from build123d import *

# Parameters (mm, degrees)
HEX_2_DEPTH = 4.7


with BuildPart() as part:
    # BodySketch → BaseBody (revolve)
    with BuildSketch(Plane(origin=(0, 0, 0), x_dir=(1, 0, 0), z_dir=(0, 1, 0)), mode=Mode.PRIVATE) as basebody_sk:
        Polygon((79.3095, 4), (80, 3.3095), (80, 0), (-0.6, 0), (-0.6, 6.5), (0, 6.5), (0, 4), align=None)
    revolve(basebody_sk.sketch.rotate(Axis((0, 0, 0), (1, 0, 0)), 180), axis=Axis((0, 0, 0), (1, 0, 0)))

    # HeadSketch → Hex 2 (add)
    with BuildSketch(Plane.ZY.offset(0.6)):
        Polygon((7.505553499, 0), (3.75277675, 6.5), (-3.75277675, 6.5), (-7.505553499, 0), (-3.75277675, -6.5), (3.75277675, -6.5), align=None)
    extrude(amount=HEX_2_DEPTH)


solid = part.part
Could you check a few things on this model? Use its own coordinates, in mm. A direction names the side the tool comes from. Coordinates: 2 decimals unless noted, no trailing zeros. Write each loop counter-clockwise with the first axis right and the second up, starting at its lowest first coordinate (ties: lowest second). Pieces come first, ordered by that corner, then holes. Notation, with made-up numbers: M -24.5,27 L 3.5,27 A21 ccw 3.5,59 Z; hole C 85,27.25 d2. An arc over 180 degrees is marked long. One line per question, with ' | ' between items.
1) I need wall thicknesses on probe 1 along X at (y, z) = (-5.25, -3); probe 2 along X at (y, z) = (-5.25, -4); probe 3 along Y at (x, z) = (4, -2). Which ranges of each line are inside material? Lowest first, please. Write a range as [from, to].
Checks:
probe 1: [-5.3, 0] | probe 2: [-5.3, -0.6] | probe 3: [-3.46, 3.46]
2) For pin 1 Ø3.5 at (y, z) = (4.5, -3) entering from +X; pin 2 Ø3 at (x, y) = (55.5, -2) entering from +Z; pin 3 Ø1.5 at (y, z) = (1.5, -6.5) entering from +X; pin 4 Ø2 at (x, z) = (50, -6) entering from -Y, each with a flat end and sliding along its axis, tell me the tip position at first contact or that it passes through.
Checks:
pin 1: x = 79.65 | pin 2: z = 3.97 | pin 3: x = 0 | pin 4: through
3) Imagine slicing it at A-A, the plane x = 69. Write out the boundary of the cut face in (y, z), and give its area (3 significant figures).
Checks:
outline: C 0,0 d8 | area: 50.3 mm²
4) For faces 1 (the face through (40.21, 3.905, -0.867)), 2 (the face through (-0.6, 6, 3)), 3 (the face through (-0.6, -6, 3)), which set-ups out of +Z, -Z, +X, -X, +Y, -Y let a thin tool reach every point of the face, with its end or its side?
Checks:
face 1: +X | face 2: +Z, +X, +Y | face 3: +Z, +X, -Y
